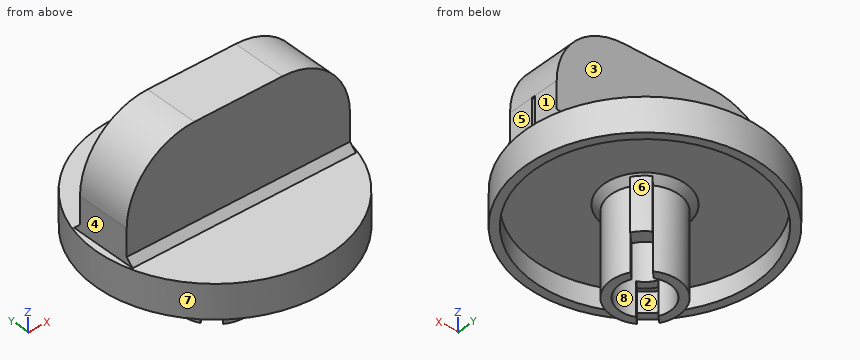
from build123d import *

# Parameters (mm, degrees)
SKETCH_R        = 17.5
PAD_DEPTH       = 5
SKETCH001_W     = 33
SKETCH001_H     = 8
PAD001_DEPTH    = 20
FILLET_R        = 10
CHAMFER_SIZE    = 1
SKETCH002_R     = 16.25
POCKET_DEPTH    = 3
SKETCH003_R     = 5
SKETCH003_R_2   = 3.75
PAD002_DEPTH    = 13
CHAMFER001_SIZE = 1
POCKET001_DEPTH = 5
PAD003_DEPTH    = 8
SKETCH006_W     = 0.5
SKETCH006_H     = 5
POCKET002_DEPTH = 1


with BuildPart() as part:
    # Sketch → Pad (new body)
    with BuildSketch(Plane.XY):
        Circle(SKETCH_R)
    extrude(amount=PAD_DEPTH)

    # Sketch001 → Pad001 (join)
    with BuildSketch(Plane.XY):
        Rectangle(SKETCH001_W, SKETCH001_H)
    extrude(amount=PAD001_DEPTH)

    # Fillet
    fillet_edges = [part.edges().sort_by_distance(p)[0] for p in [
        (-16.5, 0, 20),
        (16.5, 0, 20),
    ]]
    fillet(fillet_edges, radius=FILLET_R)

    # Chamfer
    chamfer_edges = [part.edges().sort_by_distance(p)[0] for p in [
        (0, -4, 5),
        (0, 4, 5),
    ]]
    chamfer(chamfer_edges, length=CHAMFER_SIZE)

    # Sketch002 (on Face12 of Chamfer) → Pocket (cut)
    with BuildSketch(Plane(origin=(0, 0, 0), x_dir=(1, 0, 0), z_dir=(0, 0, -1))):
        Circle(SKETCH002_R)
    extrude(amount=-POCKET_DEPTH, mode=Mode.SUBTRACT)

    # Sketch003 (on Face16 of Pocket) → Pad002 (join)
    with BuildSketch(Plane(origin=(0, 0, 3), x_dir=(1, 0, 0), z_dir=(0, 0, -1))):
        Circle(SKETCH003_R)
        Circle(SKETCH003_R_2, mode=Mode.SUBTRACT)
    extrude(amount=PAD002_DEPTH)

    # Chamfer001
    chamfer001_edges = [part.edges().sort_by_distance(p)[0] for p in [
        (-5, 0, 3),
    ]]
    chamfer(chamfer001_edges, length=CHAMFER001_SIZE)

    # Sketch004 (on Face8 of Chamfer001) → Pocket001 (cut)
    with BuildSketch(Plane(origin=(0, 0, -10), x_dir=(1, 0, 0), z_dir=(0, 0, -1))):
        Polygon((-3.071599, 4.843548), (4.621057, -2.849107), (2.85329, -4.616874), (-4.839366, 3.075782), align=None)
    extrude(amount=-POCKET001_DEPTH, mode=Mode.SUBTRACT)

    # Sketch005 (on Face10 of Pocket001) → Pad003 (join)
    with BuildSketch(Plane(origin=(0, 0, -5), x_dir=(1, 0, 0), z_dir=(0, 0, -1))):
        with BuildLine():
            ThreePointArc((3.089579, -4.849433), (4.069086, -4.062639), (4.854326, -3.081886))
            Line((4.3087, -2.53675), (4.854326, -3.081886))
            ThreePointArc((2.542013, -4.305597), (3.537693, -3.533373), (4.3087, -2.53675))
            Line((2.542013, -4.305597), (3.089579, -4.849433))
        make_face()
    extrude(amount=-PAD003_DEPTH)

    # Sketch006 (on Face27 of Pad003) → Pocket002 (cut)
    with BuildSketch(Plane.YZ.offset(16.5)):
        with Locations((0, 7.5)):
            Rectangle(SKETCH006_W, SKETCH006_H)
    extrude(amount=-POCKET002_DEPTH, mode=Mode.SUBTRACT)


solid = part.part
The model under review builds one solid part; all positions refer to its coordinate system, in mm. Face numbers are marked on the shaded views. A direction names the side the tool comes from. Give positions to 0.01 mm unless a question says otherwise; leave off trailing zeros. Order: outer loops, then holes, each group sorted by start corner. A loop starts at its lowest first (then second) coordinate and runs counter-clockwise, first axis right, second up. Notation, with made-up numbers: M 6.25,56.25 L 42.25,56.25 A24 ccw 42.25,67.25 Z; hole C 87.25,61.25 d10. An arc over 180 degrees is marked long. Answer in a Markdown table with one row per item. Add a question column.
1. Add section C-C on x = 0. State the section outline as (y, z) points, plus the area to 3 significant figures.
2. Add section D-D on y = 13. State the section outline as (x, z) points, plus the area to 3 significant figures.
3. Mouldability with a two-part tool opening along Y and no side actions: class the marked faces 5, 6, 7 and 8 as released by +Y, released by -Y, zero draft, split by the parting line, or undercut.
4. To check wall thickness, follow line 1 along Y through (x, z) = (0, 0.65); line 2 along X through (y, z) = (0, -1.25); line 3 along Z through (x, y) = (-3, 1). State the ranges of each line that lie inside material, in increasing order.
5. Machinability: for the marked faces 1, 2, 3 and 4, which of the approach directions +Z, -Z, +X, -X, +Y, -Y give a long, thin tool a straight path to every point of the face, cutting with its end or side? Answer none if there is none.
6. For pin 1 Ø4 at (y, z) = (0, 8) entering from -X; pin 2 Ø0.8 at (x, z) = (16, 7.5) entering from -Y; pin 3 Ø8 at (x, z) = (-9.5, 6) entering from -Y; pin 4 Ø5 at (y, z) = (7.5, 17) entering from +X (3 decimals), all flat-tipped, find the tip position at first contact; note any pin that passes through.
7. Add section A-A on z = 1.25. State the section outline as (x, y) points.
8. Add section B-B on z = -7.75. State the section outline as (x, y) points.
The answers:
| question | item | result |
|---|---|---|
| 1 | outline | M -17.5,0 L -16.25,0 L -16.25,3 L -6,3 L -5,2 L -5,-10 L -3.75,-10 L -3.75,3 L 3.75,3 L 3.75,-10 L 5,-10 L 5,2 L 6,3 L 16.25,3 L 16.25,0 L 17.5,0 L 17.5,5 L 5,5 L 4,6 L 4,20 L -4,20 L -4,6 L -5,5 L -17.5,5 Z |
| 1 | area | 232 mm2 |
| 2 | outline | M -11.72,0 L -9.75,0 L -9.75,3 L 9.75,3 L 9.75,0 L 11.72,0 L 11.72,5 L -11.72,5 Z |
| 2 | area | 58.7 mm2 |
| 3 | face 5 | zero draft |
| 3 | face 6 | undercut |
| 3 | face 7 | split by the parting line |
| 3 | face 8 | undercut |
| 4 | line 1 | -17.5 to -16.25, -5 to -3.75, 3.75 to 5, 16.25 to 17.5 |
| 4 | line 2 | -5 to -3.75, 3.75 to 5 |
| 4 | line 3 | 3 to 20 |
| 5 | face 1 | +Z, +X, +Y, -Y |
| 5 | face 2 | -Z |
| 5 | face 3 | +Z, +X, -X, +Y |
| 5 | face 4 | +Z, -X, +Y, -Y |
| 6 | pin 1 | x = -16.5 |
| 6 | pin 2 | y = -4 |
| 6 | pin 3 | y = -16.57 |
| 6 | pin 4 | through |
| 7 | outline | C 0,0 d35; M 2.54,4.31 A5 ccw long 4.31,2.54 L 4.85,3.08 A5.75 ccw 3.09,4.85 Z; hole C 0,0 d32.5; hole C 0,0 d7.5 |
| 8 | outline | M -4.31,-2.54 L -3.38,-1.62 A3.75 cw 1.62,3.38 L 2.54,4.31 A5 ccw Z; M -2.54,-4.31 A5 ccw 4.31,2.54 L 3.39,1.61 A3.75 cw -1.61,-3.39 Z |
